Here's how the part is built. I have some questions about the finished solid (model axes, mm). A direction names the side the tool comes from. Coordinates: 2 decimals unless noted, no trailing zeros. Write each loop counter-clockwise with the first axis right and the second up, starting at its lowest first coordinate (ties: lowest second). Pieces come first, ordered by that corner, then holes. Notation, with made-up numbers: M -15.75,-29.5 L 21.25,-29.5 A12 ccw 21.25,-14.5 Z; hole C 71.5,7.5 d6. An arc over 180 degrees is marked long. Use one line per item in the form item = value. Start each with the question number.
1. On a 3-axis mill with a long thin cutter (end or side, diameter ignored), from which of +Z, -Z, +X, -X, +Y, -Y can I reach the whole of each face in a straight line? I mean faces 5 (the face through (-3.501, -15.766, 7.888)), 6 (the face through (-6.468, -4.959, 19.465)), 7 (the face through (8, -4, 22)). Say none if no direction works.
2. Please list where these lines run through material, in increasing order: line 1 along Y through (x, z) = (0, 16.55); line 2 along Y through (x, z) = (0, 8); line 3 along X through (y, z) = (-7, 19). Write a range as [from, to].
3. I want a section at C-C, the plane z = 11.25. List the corners of the cut face in (x, y) for me.
4. Thinking about a two-plate mould opening in X: for faces 1 (the face through (1, 17, 0)), 2 (the face through (-3, -7, 16)), 3 (the face through (-4, 6, 17)), 4 (the face through (-4.01, -18.06, 10.85)), which applies, released by +X, released by -X, zero draft, split by the parting line, or undercut?
5. I want a section at D-D, the plane x = 9. List the corners of the cut face in (y, z) for me, plus the area to 3 significant figures.
6. I'm going to push flat-ended pins straight in: pin 1 Ø6 at (x, y) = (2, 3.5) entering from -Z; pin 2 Ø3 at (x, z) = (-10, 11.5) entering from -Y; pin 3 Ø5 at (x, y) = (2, -14) entering from -Z; pin 4 Ø1 at (x, z) = (-5.5, 13.5) entering from -Y. Where does each tip first touch, or does it pass through?
7. I want a section at A-A, the plane x = 0. List the corners of the cut face in (y, z) for me.
from build123d import *

# Parameters (mm, degrees)
CROQUIS1_R              = 18.5
CROQUIS1_R_2            = 16.15
SALIENTE_EXTRUIR1_DEPTH = 22
SALIENTE_EXTRUIR2_START = -5
CROQUIS2_R              = 16.15
CROQUIS2_R_2            = 8.15
SALIENTE_EXTRUIR2_DEPTH = 5
SALIENTE_EXTRUIR3_START = 1
CROQUIS3_R              = 16.15
CROQUIS3_R_2            = 7
SALIENTE_EXTRUIR3_DEPTH = 1


with BuildPart() as part:
    # Croquis1 → Saliente-Extruir1 (new body)
    with BuildSketch(Plane.XY):
        Circle(CROQUIS1_R)
        Circle(CROQUIS1_R_2, mode=Mode.SUBTRACT)
    extrude(amount=SALIENTE_EXTRUIR1_DEPTH)

    # Croquis2 → Saliente-Extruir2 (add)
    with BuildSketch(Plane.XY.offset(22).offset(SALIENTE_EXTRUIR2_START)):
        Circle(CROQUIS2_R)
        Circle(CROQUIS2_R_2, mode=Mode.SUBTRACT)
    extrude(amount=SALIENTE_EXTRUIR2_DEPTH)

    # Croquis3 → Saliente-Extruir3 (add)
    with BuildSketch(Plane(origin=(0, 0, 17), x_dir=(-1, 0, 0), z_dir=(0, 0, -1)).offset(SALIENTE_EXTRUIR3_START)):
        Circle(CROQUIS3_R)
        Circle(CROQUIS3_R_2, mode=Mode.SUBTRACT)
    extrude(amount=-SALIENTE_EXTRUIR3_DEPTH)


solid = part.part
Answer list:
q1.face_5 = -Z
q1.face_6 = +Z
q1.face_7 = +Z, +X, -X, +Y, -Y
q2.line_1 = [-18.5, -7], [7, 18.5]
q2.line_2 = [-18.5, -16.15], [16.15, 18.5]
q2.line_3 = [-17.12, -4.17], [4.17, 17.12]
q3.outline = C 0,0 d37; hole C 0,0 d32.3
q4.face_1 = zero draft
q4.face_2 = undercut
q4.face_3 = undercut
q4.face_4 = split by the parting line
q5.outline = M -16.16,0 L -13.41,0 L -13.41,16 L 13.41,16 L 13.41,0 L 16.16,0 L 16.16,22 L -16.16,22 Z
q5.area = 282 mm²
q6.pin_1 = 16
q6.pin_2 = -16.43
q6.pin_3 = 0
q6.pin_4 = -17.81
q7.outline = M -18.5,0 L -16.15,0 L -16.15,16 L -7,16 L -7,17 L -8.15,17 L -8.15,22 L -18.5,22 Z; M 7,16 L 16.15,16 L 16.15,0 L 18.5,0 L 18.5,22 L 8.15,22 L 8.15,17 L 7,17 Z
